The listing builds one solid part. Answer for the finished solid, in the listing's coordinates (mm). Face numbers are marked on the shaded views. A direction names the side the tool comes from. Round coordinates to 2 decimals unless told otherwise and drop trailing zeros. Loops run counter-clockwise (first coordinate to the right, second up) from the corner with the lowest first, then second, coordinate; pieces in that order, holes last. Notation, with made-up numbers: M 16,-22.5 L 68,-22.5 A17 cw 68,-0.5 Z; hole C 74,-3.5 d3. An arc over 180 degrees is marked long. Put each result on its own line as item: value. Start each with the question number.
(1) Section A-A, the plane z = 1.5 is taken. Determine the outline of the cut face in (x, y).
(2) Section B-B, the plane y = 0 is taken. Determine the outline of the cut face in (x, z).
(3) Section C-C, the plane x = 6.5 is taken. Determine the outline of the cut face in (y, z).
(4) Flat-ended cylindrical pins translate along their axes: P1, Ø4.5, axis at x = -23, z = 3, coming from the -Y side; P2, Ø3, axis at x = -21.5, z = 1.5, coming from the +Y side; P3, Ø10, axis at x = -22.5, y = 3, coming from the +Z side. Find the tip coordinate at first contact, or state that the pin passes through.
(5) Which of the six approach directions +Z, -Z, +X, -X, +Y, -Y give full straight-line access (tool end or side, diameter ignored) to the marked faces 1 and 2?
(6) Determine the mould class of the marked faces 3, 4 and 5 for opening direction X: released by +X, released by -X, zero draft, split by the parting line, or undercut.
(7) Straight lines are drawn through the part: line 1 (Y direction, x = -25, z = 2.65); line 2 (X direction, y = -10, z = 2.75); line 3 (X direction, y = 8.5, z = 0.25). For each, find the intervals that lie inside material, in ascending order.
(8) Section D-D, the plane z = 6.5 is taken. Determine the outline of the cut face in (x, y).
```python
from build123d import *

# Parameters (mm, degrees)
BEARING_HOUSING_PROFILE_R                  = 17
BEARING_HOUSING_PROFILE_R_2                = 11.1
BEARING_HOUSING_DEPTH                      = 7
MOUNTING_WEB_PROFILE_W                     = 30
MOUNTING_WEB_PROFILE_H                     = 28
MOUNTING_WEB_DEPTH                         = 4
BEARING_SEAT_START                         = -50
BEARING_SEAT_PROFILE_R                     = 11.1
BEARING_SEAT_DEPTH                         = 86.185224172
INNER_OUTER_RACE_RETAINING_LIP_START       = -1
INNER_OUTER_RACE_RETAINING_LIP_PROFILE_R   = 17
INNER_OUTER_RACE_RETAINING_LIP_PROFILE_R_2 = 9
INNER_OUTER_RACE_RETAINING_LIP_DEPTH       = 1
STANDOFF_FASTENERS_START                   = -50
STANDOFF_FASTENERS_PROFILE_R               = 1.6
STANDOFF_FASTENERS_DEPTH                   = 86.185224172
BEARING_KEEPER_FASTENERS_START             = -50
BEARING_KEEPER_FASTENERS_PROFILE_R         = 1.1
BEARING_KEEPER_FASTENERS_DEPTH             = 86.185224172


with BuildPart() as part:
    # Bearing_housing_profile → Bearing_housing (new body)
    with BuildSketch(Plane.XY):
        Circle(BEARING_HOUSING_PROFILE_R)
        Circle(BEARING_HOUSING_PROFILE_R_2, mode=Mode.SUBTRACT)
    extrude(amount=BEARING_HOUSING_DEPTH)

    # Mounting_web_profile → Mounting_web (add)
    with BuildSketch(Plane.XY):
        with Locations((-15, 0)):
            Rectangle(MOUNTING_WEB_PROFILE_W, MOUNTING_WEB_PROFILE_H)
    extrude(amount=MOUNTING_WEB_DEPTH)

    # Bearing_seat_profile → Bearing_seat (cut, through all)
    with BuildSketch(Plane.XY.offset(BEARING_SEAT_START)):
        Circle(BEARING_SEAT_PROFILE_R)
    extrude(amount=BEARING_SEAT_DEPTH, mode=Mode.SUBTRACT)

    # Inner_outer_race_retaining_lip_profile → Inner_outer_race_retaining_lip (add)
    with BuildSketch(Plane.XY.offset(INNER_OUTER_RACE_RETAINING_LIP_START)):
        Circle(INNER_OUTER_RACE_RETAINING_LIP_PROFILE_R)
        Circle(INNER_OUTER_RACE_RETAINING_LIP_PROFILE_R_2, mode=Mode.SUBTRACT)
    extrude(amount=INNER_OUTER_RACE_RETAINING_LIP_DEPTH)

    # Standoff_fasteners_profile → Standoff_fasteners (cut, through all)
    with BuildSketch(Plane.XY.offset(STANDOFF_FASTENERS_START)):
        with Locations(Location((-25, -9, 0), (0, 0, 180))):
            Circle(STANDOFF_FASTENERS_PROFILE_R)
        with Locations(Location((-25, 9, 0), (0, 0, 180))):
            Circle(STANDOFF_FASTENERS_PROFILE_R)
    extrude(amount=STANDOFF_FASTENERS_DEPTH, mode=Mode.SUBTRACT)

    # Bearing_keeper_fasteners_profile → Bearing_keeper_fasteners (cut, through all)
    with BuildSketch(Plane.XY.offset(BEARING_KEEPER_FASTENERS_START)):
        with Locations(Location((14, 0, 0), (0, 0, 180))):
            Circle(BEARING_KEEPER_FASTENERS_PROFILE_R)
        with Locations(Location((0, -14, 0), (0, 0, 180))):
            Circle(BEARING_KEEPER_FASTENERS_PROFILE_R)
        with Locations(Location((0, 14, 0), (0, 0, 180))):
            Circle(BEARING_KEEPER_FASTENERS_PROFILE_R)
    extrude(amount=BEARING_KEEPER_FASTENERS_DEPTH, mode=Mode.SUBTRACT)


solid = part.part
```
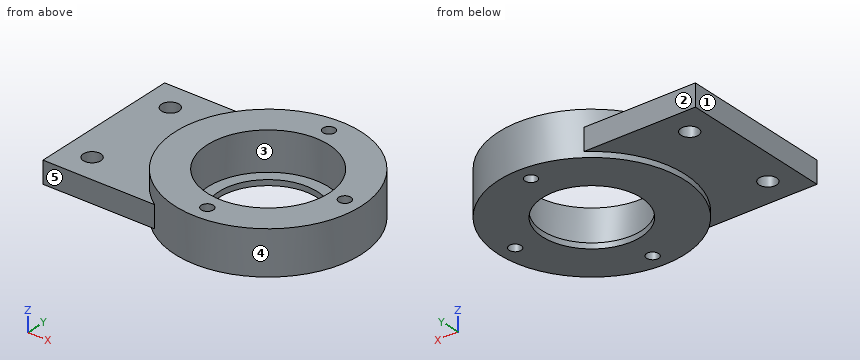
Recorded:
1. outline: M -30,-14 L -9.64,-14 A17 ccw long -9.64,14 L -30,14 Z; hole C -25,-9 d3.2; hole C -25,9 d3.2; hole C 0,0 d22.2; hole C 0,-14 d2.2; hole C 0,14 d2.2; hole C 14,0 d2.2
2. outline: M -30,0 L -17,0 L -17,-1 L -9,-1 L -9,0 L -11.1,0 L -11.1,7 L -17,7 L -17,4 L -30,4 Z; M 9,-1 L 12.9,-1 L 12.9,7 L 11.1,7 L 11.1,0 L 9,0 Z; M 15.1,-1 L 17,-1 L 17,7 L 15.1,7 Z
3. outline: M -15.71,-1 L -6.22,-1 L -6.22,0 L -9,0 L -9,7 L -15.71,7 Z; M 6.22,-1 L 15.71,-1 L 15.71,7 L 9,7 L 9,0 L 6.22,0 Z
4. P1: stops at y = -14
4. P2: stops at y = 14
4. P3: stops at z = 4
5. face 1: +Z, -Z, -X, +Y, -Y
5. face 2: +Z, -Z, -X, +Y
6. face 3: undercut
6. face 4: split by the parting line
6. face 5: zero draft
7. line 1: y = -14 to -10.6, -7.4 to 7.4, 10.6 to 14
7. line 2: x = -30 to -26.25, -23.75 to -4.82, 4.82 to 13.75
7. line 3: x = -30 to -26.52, -23.48 to -7.14, 7.14 to 14.72
8. outline: C 0,0 d34; hole C 0,0 d22.2; hole C 0,-14 d2.2; hole C 0,14 d2.2; hole C 14,0 d2.2
